Study the drawing (mm; zero at the part's minimum x, y, z) and answer. A direction names the side the tool comes from. Round coordinates to 2 decimals unless told otherwise and drop trailing zeros. Order: outer loops, then holes, each group sorted by start corner. A loop starts at its lowest first (then second) coordinate and runs counter-clockwise, first axis right, second up. Notation, with made-up numbers: (2.5, 85.5) -> (15.5, 85.5) arc R20 cw to (15.5, 115.5) -> close; hole circle Ø2 at (23, -27.75). An arc over 180 degrees is marked (long way). Use one line per item in the form item = value.
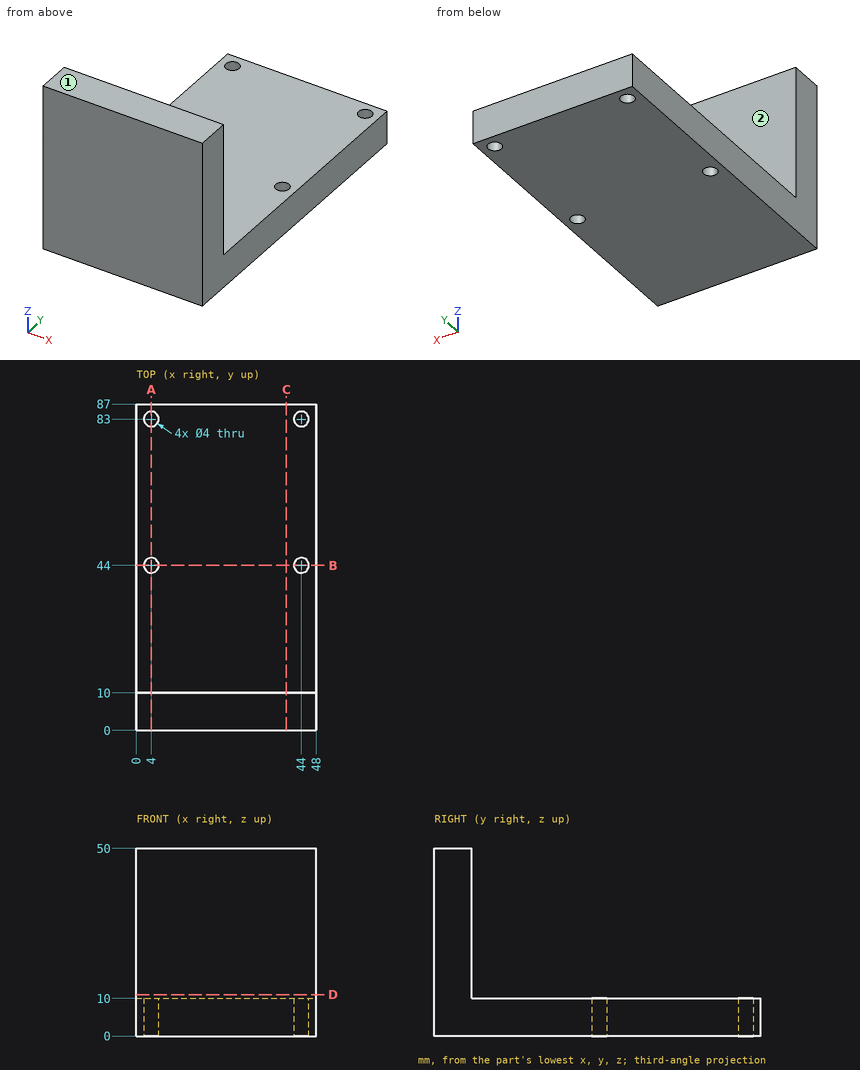
Item 1: The part is cut by section D-D, the plane z = 11. Give the vertices of the cut face in (x, y).
Findings:
outline = (0, 0) -> (48, 0) -> (48, 10) -> (0, 10) -> close
Item 2: Consider line 1 along Y through (x, z) = (4, 4.5); line 2 along X through (y, z) = (83, 6); line 3 along Y through (x, z) = (5, 11). Determine where each line is inside the solid, lowest interval first.
Findings:
line_1 = 0 to 42, 46 to 81, 85 to 87
line_2 = 0 to 2, 6 to 42, 46 to 48
line_3 = 0 to 10
Item 3: Flat-ended cylindrical pins translate along their axes: P1, Ø14.5, axis at x = 19, y = 56.5, coming from the +Z side; P2, Ø5, axis at x = 41, z = 18.5, coming from the +Y side. Find the tip coordinate at first contact, or state that the pin passes through.
Findings:
P1 = 10
P2 = 10
Item 4: The part is cut by section A-A, the plane x = 4. Give the vertices of the cut face in (y, z), and give its area (3 significant figures).
Findings:
outline = (0, 0) -> (42, 0) -> (42, 10) -> (10, 10) -> (10, 50) -> (0, 50) -> close; (46, 0) -> (81, 0) -> (81, 10) -> (46, 10) -> close; (85, 0) -> (87, 0) -> (87, 10) -> (85, 10) -> close
area = 1,190 mm^2
Item 5: The part is cut by section C-C, the plane x = 40. Give the vertices of the cut face in (y, z), and give its area (3 significant figures).
Findings:
outline = (0, 0) -> (87, 0) -> (87, 10) -> (10, 10) -> (10, 50) -> (0, 50) -> close
area = 1,270 mm^2
Item 6: For the marked faces 1 and 2, determine the directions among +Z, -Z, +X, -X, +Y, -Y from which every point of the face is accessible in a straight line to the end or side of a thin tool.
Findings:
face_1 = +Z, +X, -X, +Y, -Y
face_2 = +Z, +X, -X, +Y
Item 7: The part is cut by section B-B, the plane y = 44. Give the vertices of the cut face in (x, z).
Findings:
outline = (0, 0) -> (2, 0) -> (2, 10) -> (0, 10) -> close; (6, 0) -> (42, 0) -> (42, 10) -> (6, 10) -> close; (46, 0) -> (48, 0) -> (48, 10) -> (46, 10) -> close
